```python
from build123d import *

# Parameters (mm, degrees)
BOSS_EXTRUDE1_DEPTH             = 10
SKETCH2_W                       = 8
SKETCH2_H                       = 4.2
CUT_EXTRUDE1_DEPTH              = 4
SKETCH3_W                       = 8
SKETCH3_H                       = 4
BOSS_EXTRUDE2_DEPTH             = 4
SKETCH4_W                       = 16
SKETCH4_H                       = 4
CUT_EXTRUDE2_DEPTH              = 157.615771875
CIRPATTERN4_COUNT               = 5
CIRPATTERN4_ANGLE               = 72
CIRPATTERN4_THE_OTHER_WAY_COUNT = 5
CIRPATTERN4_THE_OTHER_WAY_ANGLE = 72


with BuildPart() as part:
    # Sketch1 → Boss-Extrude1 (new body)
    with BuildSketch(Plane(origin=(0, 0, 0), x_dir=(1, 0, 0), z_dir=(0, 1, 0))):
        with BuildLine():
            Line((-4, 112.5), (-4, 108.426242211))
            ThreePointArc((-4, 108.426242211), (-93.963756311, 54.25), (-95.899880192, -50.74901949))
            Line((-95.899880192, -50.74901949), (-99.427857926, -52.785898385))
            Line((-99.427857926, -52.785898385), (-97.427857926, -56.25))
            Line((-97.427857926, -56.25), (-91.365680099, -52.75))
            ThreePointArc((-91.365680099, -52.75), (-91.365680099, 52.75), (0, 105.5))
            Line((0, 105.5), (0, 112.5))
            Line((0, 112.5), (-4, 112.5))
        make_face()
    extrude(amount=BOSS_EXTRUDE1_DEPTH)

    # Sketch2 → Cut-Extrude1 (cut)
    with BuildSketch(Plane(origin=(-97.427857926, 0, 56.25), x_dir=(0.4999999999999976, 0, 0.86602540378444), z_dir=(-0.8660254037844402, 0, 0.4999999999999977))):
        with Locations((0, 5)):
            Rectangle(SKETCH2_W, SKETCH2_H)
    extrude(amount=-CUT_EXTRUDE1_DEPTH, mode=Mode.SUBTRACT)

    # Sketch3 → Boss-Extrude2 (add)
    with BuildSketch(Plane(origin=(0, 0, -112.5), x_dir=(-1, 0, 0), z_dir=(0, 0, -1))):
        with Locations((0, 5)):
            Rectangle(SKETCH3_W, SKETCH3_H)
    extrude(amount=-BOSS_EXTRUDE2_DEPTH)

    # Sketch4 → Cut-Extrude2 (cut, through all)
    with BuildSketch(Plane(origin=(0, 0, 0), x_dir=(0, 0, -1), z_dir=(1, 0, 0))):
        with Locations((-8.672320837, 5)):
            Rectangle(SKETCH4_W, SKETCH4_H)
    cut_extrude2 = extrude(amount=-CUT_EXTRUDE2_DEPTH, mode=Mode.SUBTRACT)

    # CirPattern4: Cut-Extrude2 ×5 about axis
    cirpattern4_axis = Axis((0, 0, 0), (0, -1, 0))
    for i in range(1, CIRPATTERN4_COUNT):
        add(cut_extrude2.rotate(cirpattern4_axis, i * CIRPATTERN4_ANGLE / (CIRPATTERN4_COUNT - 1)), mode=Mode.SUBTRACT)

    # CirPattern4 the other way: Cut-Extrude2 ×5 about axis
    cirpattern4_the_other_way_axis = Axis((0, 0, 0), (0, 1, 0))
    for i in range(1, CIRPATTERN4_THE_OTHER_WAY_COUNT):
        add(cut_extrude2.rotate(cirpattern4_the_other_way_axis, i * CIRPATTERN4_THE_OTHER_WAY_ANGLE / (CIRPATTERN4_THE_OTHER_WAY_COUNT - 1)), mode=Mode.SUBTRACT)


solid = part.part
```
The model under review builds one solid part; all positions refer to its coordinate system, in mm. A direction names the side the tool comes from. Coordinates: 2 decimals unless noted, no trailing zeros. Order: outer loops, then holes, each group sorted by start corner. A loop starts at its lowest first (then second) coordinate and runs counter-clockwise, first axis right, second up. Notation, with made-up numbers: (26, 18) -> (67, 18) arc R23 ccw to (67, 29) -> close; hole circle Ø10 at (32, 83). An arc over 180 degrees is marked (long way). Answer in a Markdown table with one row per item. Add a question column.
Item 1: Machinability: for faces 1 (the flat face through (-107, 7, 9)), 2 (the flat face through (-94.98, 5.03, 52.49)), 3 (the flat face through (2, 3, -111)), which of the approach directions +Z, -Z, +X, -X, +Y, -Y give a long, thin tool a straight path to every point of the face, cutting with its end or side? Answer none if there is none.
Item 2: We need section C-C on z = -57. Write out the cut boundary in (x, y), plus the area to 3 significant figures.
Item 3: We need section D-D on x = -21.5. Write out the cut boundary in (y, z), plus the area to 3 significant figures.
Item 4: We need section B-B on x = -46. Write out the cut boundary in (y, z), plus the area to 3 significant figures.
Item 5: We need section A-A on y = 5.5. Give the number of separate pieces and of enclosed holes in the cut face, plus the area to 3 significant figures.
Item 6: Mouldability with a two-part tool opening along Z and no side actions: class faces 4 (the flat face through (-4, 5, -110)), 5 (the flat face through (-107, 3, 9)), 6 (the flat face through (2, 5, -108.5)) as +Z half, -Z half, draft (parallel to the pull), parting line (faces both ways), or undercut.
Item 7: Clearance check with flat-ended pins moving along their axes: pin 1 (14 mm diameter, centred on x = -70, z = -84, fed in from -Y); pin 2 (1.2 mm diameter, centred on x = 1, y = 5.5, fed in from +Z); pin 3 (3 mm diameter, centred on y = 2, z = -48.5, fed in from -X); pin 4 (1 mm diameter, centred on x = -20.5, y = 8, fed in from +Z). State where each tip first meets the part, or that it passes through.
Item 8: To check wall thickness, follow probe 1 along Z at (x, y) = (-84.5, 5.5); probe 2 along Z at (x, y) = (-23, 5.25); probe 3 along X at (y, z) = (5, -46.5). State the ranges of each line that lie inside material, in increasing order.
Final values:
| question | item | result |
|---|---|---|
| 1 | face 1 | +X, -X |
| 1 | face 2 | +Z, -X |
| 1 | face 3 | +Z, -Z, +X, -Y |
| 2 | outline | (-92.32, 0) -> (-88.78, 0) -> (-88.78, 3) -> (-92.32, 3) -> close; (-92.32, 7) -> (-88.78, 7) -> (-88.78, 10) -> (-92.32, 10) -> close |
| 2 | area | 21.3 mm2 |
| 3 | outline | (0, -106.35) -> (10, -106.35) -> (10, -103.29) -> (0, -103.29) -> close |
| 3 | area | 30.6 mm2 |
| 4 | outline | (0, -98.27) -> (3, -98.27) -> (3, -94.94) -> (0, -94.94) -> close; (7, -98.27) -> (10, -98.27) -> (10, -94.94) -> (7, -94.94) -> close |
| 4 | area | 19.9 mm2 |
| 5 | separate pieces | 7 |
| 5 | enclosed holes | 0 |
| 5 | area | 415 mm2 |
| 6 | face 4 | draft |
| 6 | face 5 | undercut |
| 6 | face 6 | +Z half |
| 7 | pin 1 | stops at y = 0 |
| 7 | pin 2 | stops at z = -108.5 |
| 7 | pin 3 | stops at x = -97.79 |
| 7 | pin 4 | stops at z = -103.39 |
| 8 | probe 1 | z = -68.06 to -63.17 |
| 8 | probe 2 | z = -106.03 to -102.96 |
| 8 | probe 3 | x = -98.03 to -94.7 |
